CAD build for the part. Positions are in the model's coordinates, mm. Face numbers are marked on the shaded views. A direction names the side the tool comes from. Coordinates: 2 decimals unless noted, no trailing zeros. Write each loop counter-clockwise with the first axis right and the second up, starting at its lowest first coordinate (ties: lowest second). Pieces come first, ordered by that corner, then holes. Notation, with made-up numbers: M 84,17 L 98,17 A17 ccw 98,39 Z; hole C 83.25,44.5 d11. An arc over 180 degrees is marked long. Answer as CSV lines item,"result". Start each with the question number.
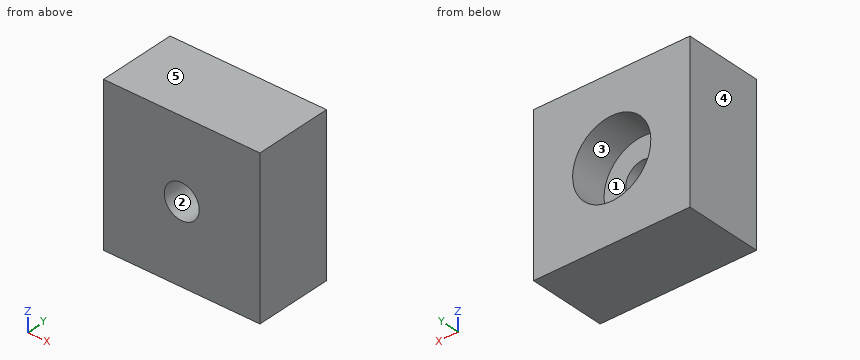
```python
from build123d import *

# Parameters (mm, degrees)
SKETCH1_W              = 38.1
SKETCH1_H              = 38.1
BOSS_EXTRUDE1_DEPTH    = 19.05
M10X1_5_TAPPED_HOLE1_D = 8.5
SKETCH5_R              = 9.525
CUT_EXTRUDE1_DEPTH     = 9


with BuildPart() as part:
    # Sketch1 → Boss-Extrude1 (new body)
    with BuildSketch(Plane(origin=(0, 0, 0), x_dir=(1, 0, 0), z_dir=(0, 1, 0))):
        Rectangle(SKETCH1_W, SKETCH1_H)
    extrude(amount=BOSS_EXTRUDE1_DEPTH)

    # M10x1.5 Tapped Hole1 (through all)
    with Locations(Plane(origin=(0, 19.05, 0), x_dir=(1, 0, 0), z_dir=(0, 1, 0))):
        with Locations((0, 0)):
            Hole(M10X1_5_TAPPED_HOLE1_D / 2)

    # Sketch5 → Cut-Extrude1 (cut)
    with BuildSketch(Plane(origin=(0, 19.05, 0), x_dir=(1, 0, 0), z_dir=(0, 1, 0))):
        with Locations(Location((0, 0, 0), (0, 0, 270))):
            Circle(SKETCH5_R)
    extrude(amount=-CUT_EXTRUDE1_DEPTH, mode=Mode.SUBTRACT)


solid = part.part
```
1) Pin check, flat tips, straight feed: P1, Ø5.5, axis at x = -4, z = 3, coming from the +Y side; P2, Ø11.5, axis at x = 0, z = 0, coming from the +Y side. Stop position of each tip, or through.
2) Tool access for the marked faces 1 and 2: list every direction of +Z, -Z, +X, -X, +Y, -Y with a clear straight run to the whole face (end or side of a thin tool).
3) Probe L1, parallel to Z at x = 0, y = 7.75; L2, parallel to X at y = 15.75, z = 0 (3 decimals); L3, parallel to Y at x = -4, z = -7. List the from-to ranges inside material, lowest first. Write a range as [from, to].
4) Band-saw the part on A-A, the plane x = 0. List the corners of the cut face in (y, z) (3 decimals), plus the area to 3 significant figures.
5) Band-saw the part on D-D, the plane z = -9. List the corners of the cut face in (x, y).
6) Two-plate mould, pull along Z, no slides. Class the marked faces 3, 4 and 5: pulls with the +Z half, pulls with the -Z half, needs draft (parallel to the pull), parting line crosses it, or undercut.
7) Band-saw the part on B-B, the plane z = 0. List the corners of the cut face in (x, y) (3 decimals).
8) Band-saw the part on C-C, the plane y = 8. List the corners of the cut face in (x, z).
Result sheet:
1,P1,"stops at y = 10.05"
1,P2,"stops at y = 10.05"
2,face 1,"+Y"
2,face 2,"+Y, -Y"
3,L1,"z = [-19.05, -4.25], [4.25, 19.05]"
3,L2,"x = [-19.05, -9.525], [9.525, 19.05]"
3,L3,"y = [0, 10.05]"
4,outline,"M 0,-19.05 L 19.05,-19.05 L 19.05,-9.525 L 10.05,-9.525 L 10.05,-4.25 L 0,-4.25 Z; M 0,4.25 L 10.05,4.25 L 10.05,9.525 L 19.05,9.525 L 19.05,19.05 L 0,19.05 Z"
4,area,"469 mm²"
5,outline,"M -19.05,0 L 19.05,0 L 19.05,19.05 L 3.12,19.05 L 3.12,10.05 L -3.12,10.05 L -3.12,19.05 L -19.05,19.05 Z"
6,face 3,"undercut"
6,face 4,"needs draft"
6,face 5,"pulls with the +Z half"
7,outline,"M -19.05,0 L -4.25,0 L -4.25,10.05 L -9.525,10.05 L -9.525,19.05 L -19.05,19.05 Z; M 4.25,0 L 19.05,0 L 19.05,19.05 L 9.525,19.05 L 9.525,10.05 L 4.25,10.05 Z"
8,outline,"M -19.05,-19.05 L 19.05,-19.05 L 19.05,19.05 L -19.05,19.05 Z; hole C 0,0 d8.5"
